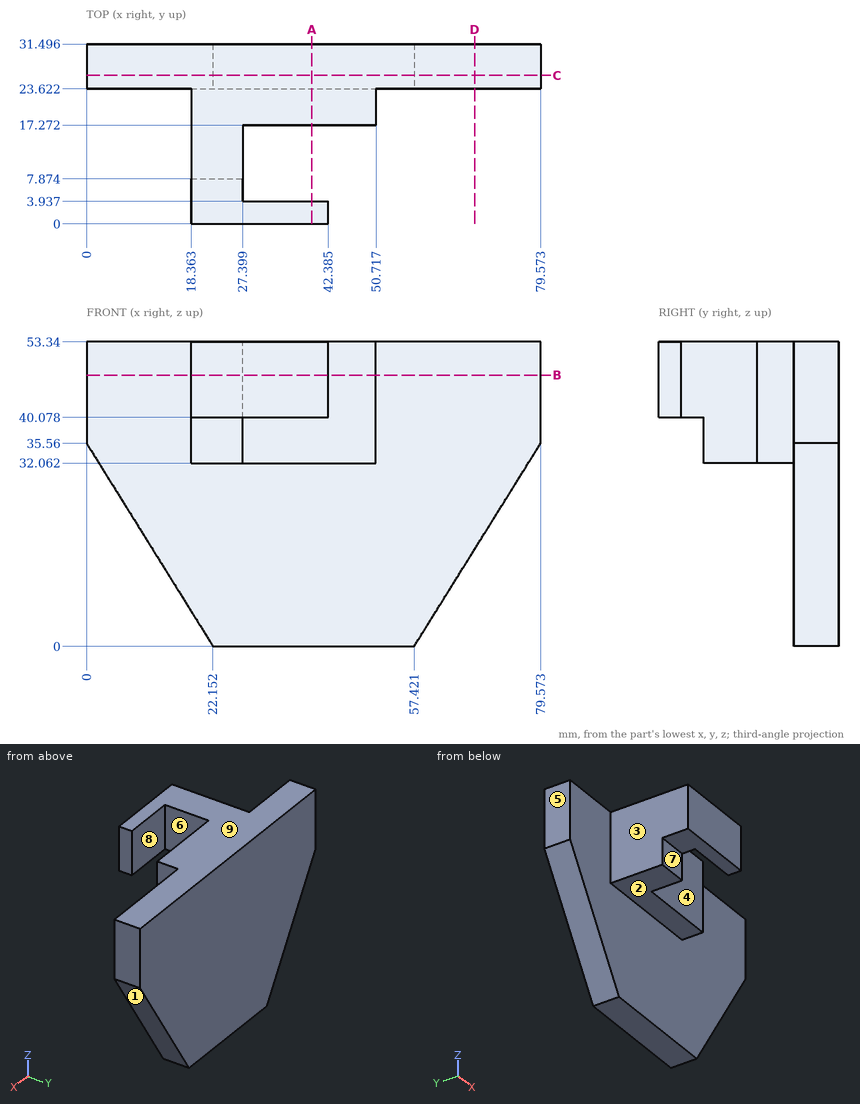
Geometry check sheet. Reference: drawing and pictorial views, mm from the part's lowest x, y, z. A direction names the side the tool comes from. Coordinates: 2 decimals unless noted, no trailing zeros. Order: outer loops, then holes, each group sorted by start corner. A loop starts at its lowest first (then second) coordinate and runs counter-clockwise, first axis right, second up. Notation, with made-up numbers: (79, 59) - (109, 59) arc R19 cw to (109, 96) - close; hole circle Ø4 at (-29.75, 46). An arc over 180 degrees is marked (long way). Answer in a Markdown table with one row per item. Add a question column.
1) Release check for a two-part mould opening along Y. For the marked faces 6, 7, 8 and 9 record: +Y half, -Y half, draft (parallel to the pull), parting line (faces both ways), or undercut.
2) Cross-section at D-D, the plane x = 68. Record the cut outline in (y, z).
3) Set-up check for the marked faces 1, 2, 3, 4 and 5: record each of +Z, -Z, +X, -X, +Y, -Y from which the full face is reachable in a straight line by a thin tool's end or side.
4) Cross-section at B-B, the plane z = 47.5. Record the cut outline in (x, y) (1 decimal).
5) Cross-section at A-A, the plane x = 39.5. Record the cut outline in (y, z).
6) Gauge pin test, flat ends, axial feed: P1, Ø10, axis at y = 27.5, z = 12, coming from the +X side; P2, Ø4.5, axis at y = 1.5, z = 44.5, coming from the +X side (1 decimal); P3, Ø3, axis at y = 21.5, z = 38.5, coming from the +X side. Record the tip position at first contact, or that the pin passes through.
7) Cross-section at C-C, the plane y = 26. Record the cut outline in (x, z), then the cut area to 3 significant figures.
8) Material ranges on line 1 along Y through (x, z) = (12.5, 40); line 2 along X through (y, z) = (21.5, 36.5); line 3 along Y through (x, z) = (19, 33), recorded low to high. Write a range as [from, to].
Check result:
| question | item | result |
|---|---|---|
| 1 | face 6 | undercut |
| 1 | face 7 | -Y half |
| 1 | face 8 | undercut |
| 1 | face 9 | draft |
| 2 | outline | (23.62, 16.98) - (31.5, 16.98) - (31.5, 53.34) - (23.62, 53.34) - close |
| 3 | face 1 | -Z, +X, +Y, -Y |
| 3 | face 2 | -Z, +X, -X, -Y |
| 3 | face 3 | +Z, -Z, -X, -Y |
| 3 | face 4 | +Z, -Z, +X |
| 3 | face 5 | +Z, -Z, -X, +Y, -Y |
| 4 | outline | (0, 23.6) - (18.4, 23.6) - (18.4, 0) - (42.4, 0) - (42.4, 3.9) - (27.4, 3.9) - (27.4, 17.3) - (50.7, 17.3) - (50.7, 23.6) - (79.6, 23.6) - (79.6, 31.5) - (0, 31.5) - close |
| 5 | outline | (0, 40.08) - (3.94, 40.08) - (3.94, 53.34) - (0, 53.34) - close; (17.27, 32.06) - (23.62, 32.06) - (23.62, 0) - (31.5, 0) - (31.5, 53.34) - (17.27, 53.34) - close |
| 6 | P1 | stops at x = 68.01 |
| 6 | P2 | stops at x = 42.4 |
| 6 | P3 | stops at x = 50.72 |
| 7 | outline | (0, 35.56) - (22.15, 0) - (57.42, 0) - (79.57, 35.56) - (79.57, 53.34) - (0, 53.34) - close |
| 7 | area | 3,460 mm² |
| 8 | line 1 | y = [23.62, 31.5] |
| 8 | line 2 | x = [18.36, 50.72] |
| 8 | line 3 | y = [7.87, 31.5] |
